Source: CAD feature listing. Evaluate the final solid. Frame: model axes, mm. Face numbers are marked on the shaded views. A direction names the side the tool comes from. Give positions to 0.01 mm unless a question says otherwise; leave off trailing zeros. Loops run counter-clockwise (first coordinate to the right, second up) from the corner with the lowest first, then second, coordinate; pieces in that order, holes last.
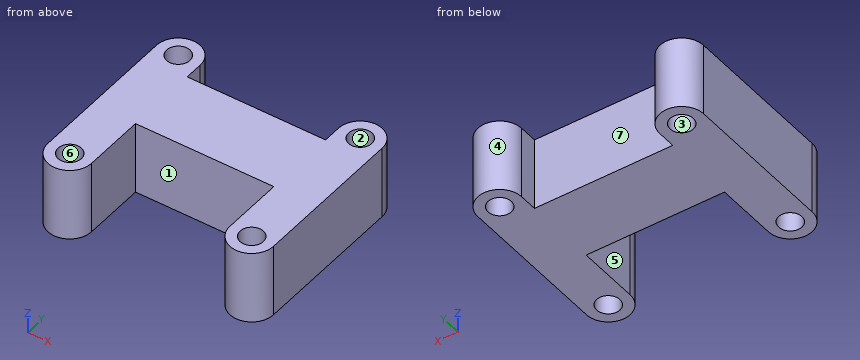
```python
from build123d import *

# Parameters (mm, degrees)
SKETCH1_R           = 1.6
SKETCH1_W           = 19
SKETCH1_H           = 10
BOSS_EXTRUDE1_DEPTH = 10


with BuildPart() as part:
    # Sketch1 → Boss-Extrude1 (new body)
    with BuildSketch(Plane.XY):
        with BuildLine():
            Line((3, 0), (3, 21))
            ThreePointArc((3, 21), (0, 24), (-3, 21))
            Line((-3, 21), (-3, 0))
            ThreePointArc((-3, 0), (0, -3), (3, 0))
        make_face()
        Circle(SKETCH1_R, mode=Mode.SUBTRACT)
        with Locations((0, 21)):
            Circle(SKETCH1_R, mode=Mode.SUBTRACT)
        with Locations((12.5, 13.5)):
            Rectangle(SKETCH1_W, SKETCH1_H)
        with BuildLine():
            Line((22, 18.5), (22, 8.5))
            Line((22, 8.5), (22, 0))
            ThreePointArc((22, 0), (25, -3), (28, 0))
            Line((28, 0), (28, 21))
            ThreePointArc((28, 21), (25, 24), (22, 21))
            Line((22, 21), (22, 18.5))
        make_face()
        with Locations((25, 0)):
            Circle(SKETCH1_R, mode=Mode.SUBTRACT)
        with Locations((25, 21)):
            Circle(SKETCH1_R, mode=Mode.SUBTRACT)
    extrude(amount=BOSS_EXTRUDE1_DEPTH)


solid = part.part
```
(1) Reachability of the marked faces 5, 6 and 7 from +Z, -Z, +X, -X, +Y, -Y: full face, straight path, thin tool, end or side. Return the list, or none.
A:
face 5: +Z, -Z, -Y
face 6: +Z, -Z
face 7: +Z, -Z, +Y
(2) Section A-A, the plane x = 25. Return the cut outline in (y, z), then the cut area to 3 significant figures.
A:
outline: (-3, 0) - (-1.6, 0) - (-1.6, 10) - (-3, 10) - close; (1.6, 0) - (19.4, 0) - (19.4, 10) - (1.6, 10) - close; (22.6, 0) - (24, 0) - (24, 10) - (22.6, 10) - close
area: 206 mm2
(3) First-contact query: pin 1 (1.5 mm diameter, centred on x = 3.5, z = 7.5, fed in from +Y); pin 2 (2.5 mm diameter, centred on x = 25, y = 21, fed in from +Z); pin 3 (5 mm diameter, centred on x = 9, z = 3.5, fed in from +Y); pin 4 (5 mm diameter, centred on x = 20.5, z = 5, fed in from +Y). Flat tips, straight axial feed; report the tip coordinate or a pass-through.
A:
pin 1: stops at y = 22.2
pin 2: passes through
pin 3: stops at y = 18.5
pin 4: stops at y = 23.24
(4) Ray query, line 1 along Y through (x, z) = (25, 2.5); line 2 along X through (y, z) = (7.25, 4.25); line 3 along X through (y, z) = (22, 9.25). Return the intervals inside material, ascending.
A:
line 1: y = -3 to -1.6, 1.6 to 19.4, 22.6 to 24
line 2: x = -3 to 3, 22 to 28
line 3: x = -2.83 to -1.25, 1.25 to 2.83, 22.17 to 23.75, 26.25 to 27.83
(5) Section D-D, the plane y = 0.75. Return the cut outline in (x, z), then the cut area to 3 significant figures.
A:
outline: (-3, 0) - (-1.41, 0) - (-1.41, 10) - (-3, 10) - close; (1.41, 0) - (3, 0) - (3, 10) - (1.41, 10) - close; (22, 0) - (23.59, 0) - (23.59, 10) - (22, 10) - close; (26.41, 0) - (28, 0) - (28, 10) - (26.41, 10) - close
area: 63.5 mm2
(6) Section C-C, the plane y = 5.25. Return the cut outline in (x, z).
A:
outline: (-3, 0) - (3, 0) - (3, 10) - (-3, 10) - close; (22, 0) - (28, 0) - (28, 10) - (22, 10) - close
(7) Mould query, pull axis Y, two halves, no side actions, for the marked faces 1, 2, 3 and 4. Classes: pulls with the +Y half, pulls with the -Y half, needs draft (parallel to the pull), parting line crosses it, or undercut.
A:
face 1: pulls with the -Y half
face 2: undercut
face 3: undercut
face 4: pulls with the +Y half
(8) Section B-B, the plane z = 8.5. Return the cut outline in (x, y), then the cut area to 3 significant figures.
A:
outline: (-3, 0) arc R3 ccw to (3, 0) - (3, 8.5) - (22, 8.5) - (22, 0) arc R3 ccw to (28, 0) - (28, 21) arc R3 ccw to (22, 21) - (22, 18.5) - (3, 18.5) - (3, 21) arc R3 ccw to (-3, 21) - close; hole circle Ø3.2 at (0, 0); hole circle Ø3.2 at (0, 21); hole circle Ø3.2 at (25, 0); hole circle Ø3.2 at (25, 21)
area: 466 mm2
